from build123d import *

# Parameters (mm, degrees)
SKETCH1_R           = 16.1655
BOSS_EXTRUDE1_DEPTH = 13.5
FILLET1_R           = 1
SKETCH2_R           = 12.5
SKETCH2_R_2         = 11
BOSS_EXTRUDE2_DEPTH = 1
FILLET4_R           = 0.707
SKETCH3_R           = 13.168514768
BOSS_EXTRUDE3_DEPTH = 2


with BuildPart() as part:
    # Sketch1 → Boss-Extrude1 (new body)
    with BuildSketch(Plane(origin=(0, 0, 0), x_dir=(1, 0, 0), z_dir=(0, 1, 0))):
        Circle(SKETCH1_R)
    extrude(amount=BOSS_EXTRUDE1_DEPTH)

    # Fillet1
    fillet1_edges = [part.edges().sort_by_distance(p)[0] for p in [
        (-16.1655, 0, 0),
        (-16.1655, 13.5, 0),
    ]]
    fillet(fillet1_edges, radius=FILLET1_R)

    # Sketch2 → Boss-Extrude2 (add)
    with BuildSketch(Plane(origin=(0, 13.5, 0), x_dir=(1, 0, 0), z_dir=(0, 1, 0))):
        Circle(SKETCH2_R)
        Circle(SKETCH2_R_2, mode=Mode.SUBTRACT)
    extrude(amount=BOSS_EXTRUDE2_DEPTH)

    # Fillet4
    fillet4_edges = [part.edges().sort_by_distance(p)[0] for p in [
        (-12.5, 14.5, 0),
        (-11, 14.5, 0),
    ]]
    fillet(fillet4_edges, radius=FILLET4_R)

    # Sketch3 → Boss-Extrude3 (add)
    with BuildSketch(Plane.XZ):
        Circle(SKETCH3_R)
    extrude(amount=BOSS_EXTRUDE3_DEPTH)


solid = part.part
Can you work these out from the model? Positions are in its coordinate system, mm. A direction names the side the tool comes from. Round coordinates to 2 decimals unless told otherwise and drop trailing zeros. Order: outer loops, then holes, each group sorted by start corner. A loop starts at its lowest first (then second) coordinate and runs counter-clockwise, first axis right, second up. Notation, with made-up numbers: (65.5, 77) - (89.5, 77) arc R19 cw to (89.5, 83) - close; hole circle Ø1 at (80, -27). An arc over 180 degrees is marked (long way). Answer in a Markdown table with one row per item.
(1) If we mould it in two halves opening along Z, with no side actions, what happens to faces 1 (the face through (0, 13.5, 0)), 2 (the face through (-1.714, -0.986, 13.056)), 3 (the face through (0, 0, -14))? For each: released by +Z, released by -Z, zero draft, split by the parting line, or undercut.
From the geometry:
| item | result |
|---|---|
| face 1 | undercut |
| face 2 | split by the parting line |
| face 3 | zero draft |
(2) For P1, Ø2, axis at y = 5.5, z = 1.5, coming from the -X side; P2, Ø4, axis at y = 10.5, z = -9, coming from the -X side; P3, Ø9, axis at x = 4, z = 2.5, coming from the +Y side, each with a flat end and sliding along its axis, tell me the tip position at first contact or that it passes through.
From the geometry:
| item | result |
|---|---|
| P1 | stops at x = -16.16 |
| P2 | stops at x = -14.57 |
| P3 | stops at y = 13.5 |
(3) Suppose I cut it at B-B, the plane x = 0. Please give me the cut outline in (y, z).
From the geometry:
| item | result |
|---|---|
| outline | (-2, -13.17) - (0, -13.17) - (0, -15.17) arc R1 ccw to (1, -16.17) - (12.5, -16.17) arc R1 ccw to (13.5, -15.17) - (13.5, -12.5) - (13.79, -12.5) arc R0.71 ccw to (14.5, -11.79) - (14.5, -11.71) arc R0.71 ccw to (13.79, -11) - (13.5, -11) - (13.5, 11) - (13.79, 11) arc R0.71 ccw to (14.5, 11.71) - (14.5, 11.79) arc R0.71 ccw to (13.79, 12.5) - (13.5, 12.5) - (13.5, 15.17) arc R1 ccw to (12.5, 16.17) - (1, 16.17) arc R1 ccw to (0, 15.17) - (0, 13.17) - (-2, 13.17) - close |
(4) Suppose I cut it at C-C, the plane y = 4.5. Please give me the cut outline in (x, z).
From the geometry:
| item | result |
|---|---|
| outline | circle Ø32.33 at (0, 0) |
(5) Suppose I cut it at A-A, the plane z = 0. Please give me the cut outline in (x, y), plus the area to 3 significant figures.
From the geometry:
| item | result |
|---|---|
| outline | (-16.17, 1) arc R1 ccw to (-15.17, 0) - (-13.17, 0) - (-13.17, -2) - (13.17, -2) - (13.17, 0) - (15.17, 0) arc R1 ccw to (16.17, 1) - (16.17, 12.5) arc R1 ccw to (15.17, 13.5) - (12.5, 13.5) - (12.5, 13.79) arc R0.71 ccw to (11.79, 14.5) - (11.71, 14.5) arc R0.71 ccw to (11, 13.79) - (11, 13.5) - (-11, 13.5) - (-11, 13.79) arc R0.71 ccw to (-11.71, 14.5) - (-11.79, 14.5) arc R0.71 ccw to (-12.5, 13.79) - (-12.5, 13.5) - (-15.17, 13.5) arc R1 ccw to (-16.17, 12.5) - close |
| area | 491 mm2 |
(6) Please list where these lines run through material, in increasing order: L1, parallel to Z at x = 0, y = 13.75; L2, parallel to Y at x = 12.5, z = 5.5. Write a range as from..to.
From the geometry:
| item | result |
|---|---|
| L1 | z = -12.5..-11, 11..12.5 |
| L2 | y = 0..13.5 |
(7) Which directions (+Z, -Z, +X, -X, +Y, -Y) give clear straight access to the entire face, cutting with the end or side of a thin tool? Please do faces 4 (the face through (-5.7, 13.5, -11.3)), 5 (the face through (0, -2, 0)).
From the geometry:
| item | result |
|---|---|
| face 4 | +Y |
| face 5 | +Z, -Z, +X, -X, -Y |
